from build123d import *

# Parameters (mm, degrees)
F2_W     = 5.81
F2_H     = 12.85
F3_DEPTH = 6.62
F6_DEPTH = 2.6
F7_SIZE2 = 11.84999
F7_SIZE  = 2.59999


# Not quite as in the source:
# - a fillet or chamfer is up to 0.001 mm smaller than in the source, because OpenCascade refuses the exact size


with BuildPart() as f3:
    # F2 (on Top) → F3 (new body)
    with BuildSketch(Plane.XY):
        Rectangle(F2_W, F2_H)
    extrude(amount=F3_DEPTH)

    # F4 (on face) → F6 (join)
    with BuildSketch(Plane.XY.offset(6.62)):
        Polygon((2, 5.925), (-2, 5.925), (-1.575, -5.925), (1.575, -5.925), align=None)
    extrude(amount=F6_DEPTH)

    # F7 (size 2.6 and 11.85 in the source; OpenCascade refuses exactly that, so slightly less here)
    f7_edges = [f3.edges().sort_by_distance(p)[0] for p in [
        (0, 5.925, 9.22),
    ]]
    f7_side = f3.faces().sort_by_distance((0, 5.925, 7.92))[0]
    chamfer(f7_edges, length=F7_SIZE, length2=F7_SIZE2, reference=f7_side)


solid = f3.part
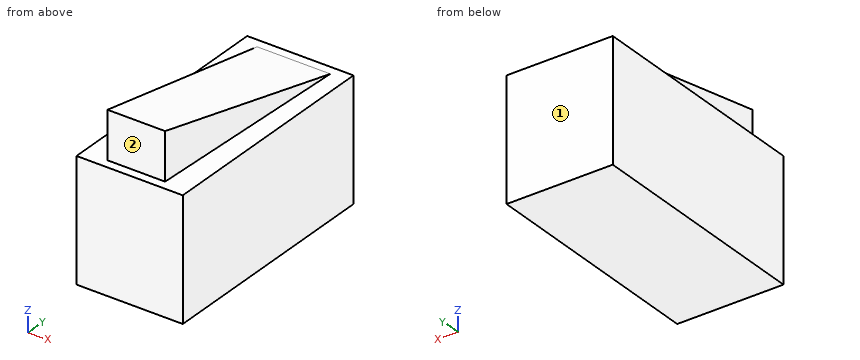
Here's how the part is built. I have some questions about the finished solid (model axes, mm). Face numbers are marked on the shaded views. A direction names the side the tool comes from. Coordinates: 2 decimals unless noted, no trailing zeros. Write each loop counter-clockwise with the first axis right and the second up, starting at its lowest first coordinate (ties: lowest second). Pieces come first, ordered by that corner, then holes.
1) Which directions (+Z, -Z, +X, -X, +Y, -Y) give clear straight access to the entire face, cutting with the end or side of a thin tool? Please do the marked faces 1 and 2.
Filled in:
face 1: +Z, -Z, +X, -X, +Y
face 2: +Z, +X, -X, -Y
2) If we section it at B-B (y = 4.25): List the corners of the cut face in (x, z) for me (3 decimals).
Filled in:
outline: (-2.905, 0) - (2.905, 0) - (2.905, 6.62) - (1.94, 6.62) - (1.94, 6.988) - (-1.94, 6.988) - (-1.94, 6.62) - (-2.905, 6.62) - close
3) If I drill on line 1 (Z direction, x = 2.15, y = -0.5); line 2 (Z direction, x = 1.75, y = 3.75); line 3 (X direction, y = -3.25, z = 7.75), over which ranges is the centre line in solid material (lowest first)?
Filled in:
line 1: z = 0 to 6.62
line 2: z = 0 to 7.1
line 3: x = -1.67 to 1.67
4) I'm going to push flat-ended pins straight in: pin 1 (2 mm diameter, centred on x = 0, z = 8.5, fed in from -Y) (3 decimals); pin 2 (3 mm diameter, centred on x = 1, y = -2, fed in from +Z); pin 3 (1.5 mm diameter, centred on x = -2, y = 0, fed in from +Z); pin 4 (1 mm diameter, centred on x = 1.5, y = 0, fed in from -Z). Where does each tip first touch, or does it pass through?
Filled in:
pin 1: stops at y = -5.925
pin 2: stops at z = 8.69
pin 3: stops at z = 8.08
pin 4: stops at z = 0
